Model file for the job. Use its own axes, mm. A direction names the side the tool comes from. Round coordinates to 2 decimals unless told otherwise and drop trailing zeros. Write each loop counter-clockwise with the first axis right and the second up, starting at its lowest first coordinate (ties: lowest second). Pieces come first, ordered by that corner, then holes. Notation, with made-up numbers: (25.25, -27.75) - (66.25, -27.75) arc R29 cw to (66.25, 6.25) - close; hole circle Ø8 at (-11.5, 3). An arc over 180 degrees is marked (long way). One line per item, written item: value.
Autodesk Inventor part; units mm, degrees
ref_plane "Arbeitsebene2" through (4.7579, -7.132, 2.2) normal (0, 0, 1) x (1, 0, 0)
ref_plane "YZ Plane" through (0, 0, 0) normal (1, 0, 0) x (0, 1, 0)
ref_plane "XZ Plane" through (0, 0, 0) normal (0, 1, 0) x (-1, 0, 0)
ref_plane "Arbeitsebene1" through (0, 0, 0) normal (0, 0, 1) x (1, 0, 0)
sketch "Skizze1" plane through (0, 0, 0) normal (0, 0, 1) x (1, 0, 0)
  circle A0 centre (-0.0001, 0.0021) radius 3
  circle A1 centre (11, 0) radius 2.566
  circle A2 centre (-9.5, -11) radius 1.352
  arc A3 (19, -13.5) -> (20, -12.5) centre (19, -12.5) ccw
  line L0 (20, -12.5) -> (20, 12.5)
  arc A4 (20, 12.5) -> (19, 13.5) centre (19, 12.5) ccw
  line L1 (19, 13.5) -> (-19, 13.5)
  arc A5 (-19, 13.5) -> (-20, 12.5) centre (-19, 12.5) ccw
  line L2 (-20, 12.5) -> (-20, -12.5)
  arc A6 (-20, -12.5) -> (-19, -13.5) centre (-19, -12.5) ccw
  line L3 (-19, -13.5) -> (19, -13.5)
  line L4 (18.6579, -7.132) -> (11.0758, -7.132)
  line L5 (18.6579, -7.132) -> (18.6579, 2.268)
  line L6 (18.6579, 2.268) -> (19.6579, 4.268)
  line L7 (19.6579, 4.268) -> (19.6579, 7.668)
  line L8 (18.0704, 7.668) -> (19.6579, 7.668)
  line L9 (18.0704, 7.668) -> (18.0704, 6.818)
  line L10 (18.0704, 6.818) -> (13.4704, 6.818)
  line L11 (13.4704, 6.818) -> (13.4704, 5.418)
  line L12 (13.4704, 5.418) -> (14.8704, 5.418)
  line L13 (14.8704, 5.418) -> (15.4704, 6.018)
  line L14 (15.4704, 6.018) -> (18.0704, 6.018)
  line L15 (18.0704, 6.018) -> (18.0704, 5.768)
  line L16 (18.0704, 5.768) -> (15.5704, 5.768)
  line L17 (15.5704, 5.768) -> (15.0704, 5.268)
  line L18 (15.0704, 5.268) -> (13.0704, 5.268)
  line L19 (13.0704, 5.268) -> (13.0704, 7.668)
  line L20 (6.4079, 7.668) -> (13.0704, 7.668)
  line L21 (6.4079, 7.668) -> (6.4079, 6.468)
  line L22 (4.7579, 6.468) -> (6.4079, 6.468)
  line L23 (4.7579, -7.132) -> (4.7579, 6.468)
  line L24 (5.4458, -7.132) -> (4.7579, -7.132)
  line L25 (5.4458, -7.132) -> (5.4458, -6.382)
  line L26 (5.4458, -6.382) -> (11.0758, -6.382)
  line L27 (11.0758, -6.382) -> (11.0758, -7.132)
  line L28 (9.0327, 10.168) -> (-5.2421, 10.168)
  line L29 (-5.2421, 10.168) -> (-5.2421, 8.168)
  line L30 (-5.2421, 8.168) -> (9.0327, 8.168)
  line L31 (9.0327, 8.168) -> (9.0327, 10.168)
  line L32 (-5.2421, 8.168) -> (4.7579, 8.168)
  line L33 (4.7579, 8.168) -> (4.7579, -9.632)
  line L34 (4.7579, -9.632) -> (-5.2421, -9.632)
  line L35 (-5.2421, -9.632) -> (-5.2421, 8.168)
  line L36 (4.7579, -9.632) -> (9.0327, -9.632)
  line L37 (9.0327, -9.632) -> (9.0327, -7.632)
  line L38 (9.0327, -7.632) -> (4.7579, -7.632)
  line L39 (4.7579, -7.632) -> (4.7579, -9.632)
  point P0 (0, 0)
  point P1 (4.7579, 8.168)
  dimension "d0" = 0
  dimension "d1" = 0.5
  dimension "d2" = 0.5
  dimension "d3" = 2
  dimension "d4" = 2
  dimension "d5" = 10
ref_plane "Arbeitsebene2" through (4.7579, -7.132, 2.2) normal (0, 0, 1) x (1, 0, 0)
extrude "Extrusion1" add sketch "Skizze1" along normal up to surface (2.2 mm away) contours A0 | L33 L34 L35 L30 L23 | L38 L37 L36 L33 | L30 L29 L28 L31
sketch "Skizze2" plane through (-5.2421, 10.168, 2.2) normal (0, 0, 1) x (1, 0, 0)
  line L0 (0, 0) -> (14.2747, 0)
  line L1 (0, -19.8) -> (0, 0)
  line L2 (14.2747, -19.8) -> (0, -19.8)
  line L3 (14.2747, -17.8) -> (14.2747, -19.8)
  line L4 (10, -17.8) -> (14.2747, -17.8)
  line L5 (10, -2) -> (10, -17.8)
  line L6 (14.2747, -2) -> (10, -2)
  line L7 (14.2747, 0) -> (14.2747, -2)
  line L8 (14.2747, 0) -> (0, 0)
  line L9 (14.2747, 0) -> (0, 0)
  line L10 (0, 0) -> (0, -19.8)
  line L11 (0, -19.8) -> (14.2747, -19.8)
  line L12 (14.2747, -19.8) -> (14.2747, 0)
  line L13 (9.6421, -14.568) -> (0.8421, -14.568)
  line L14 (0.8421, -14.568) -> (0.8421, -5.768)
  line L15 (0.8421, -5.768) -> (9.6421, -5.768)
  line L16 (9.6421, -5.768) -> (9.6421, -14.568)
  line L17 (9.6421, -14.568) -> (0.8421, -5.768) construction
  line L18 (0.8421, -14.568) -> (9.6421, -5.768) construction
  line L19 (0, 0) -> (0, -19.8)
  line L20 (0.8421, -5.768) -> (0, -5.768)
  line L21 (0, -5.768) -> (0, -14.568)
  line L22 (0, -14.568) -> (0.8421, -14.568)
  line L23 (0.8421, -14.568) -> (0.8421, -5.768)
  point P0 (5.2421, -10.168)
  point P1 (0, -5.768)
  point P2 (0.8421, -14.568)
  point P3 (14.2747, -17.8)
  point P4 (14.2747, -2)
  dimension "d8" = 8.8
  dimension "d9" = 8.8
extrude "Extrusion2" add sketch "Skizze2" along normal blind 2 contours L0 L7 L6 L5 L4 L3 L2 L1 L22 L13 L16 L15 L20 | L12 L4 L5 L6
sketch "Skizze3" plane through (0, 0, 0) normal (0, 0, -1) x (-1, 0, 0)
  line L0 (5.2421, 10.168) -> (5.2421, -9.632)
  line L1 (-9.0327, 10.168) -> (5.2421, 10.168)
  line L2 (-9.0327, 8.168) -> (-9.0327, 10.168)
  line L3 (-4.7579, 8.168) -> (-9.0327, 8.168)
  line L4 (-4.7579, -7.632) -> (-4.7579, 8.168)
  line L5 (-9.0327, -7.632) -> (-4.7579, -7.632)
  line L6 (-9.0327, -9.632) -> (-9.0327, -7.632)
  line L7 (5.2421, -9.632) -> (-9.0327, -9.632)
  line L8 (2.2421, -9.8367) -> (9.0217, -9.8367)
  line L9 (9.0217, -9.8367) -> (9.0217, 10.4786)
  line L10 (9.0217, 10.4786) -> (2.2421, 10.4786)
  line L11 (2.2421, 10.4786) -> (2.2421, -9.8367)
  line L12 (2.2421, -9.8367) -> (9.0217, 10.4786) construction
  line L13 (9.0217, -9.8367) -> (2.2421, 10.4786) construction
  point P0 (0, 0)
  point P1 (5.6319, 0.321)
  dimension "d12" = 3
extrude "Extrusion3" cut sketch "Skizze3" against normal blind 2.5 contours L1 L11 L10 L9 L8 L7 L0 | L0 L7 L11 L1
sketch "Skizze4" plane through (0, 0, 0) normal (0, 0, -1) x (-1, 0, 0)
  line L0 (2.2421, -9.632) -> (2.2421, 10.168)
  line L1 (-9.0327, 10.168) -> (2.2421, 10.168)
  line L2 (-9.0327, 8.168) -> (-9.0327, 10.168)
  line L3 (-4.7579, 8.168) -> (-9.0327, 8.168)
  line L4 (-4.7579, -7.632) -> (-4.7579, 8.168)
  line L5 (-9.0327, -7.632) -> (-4.7579, -7.632)
  line L6 (-9.0327, -9.632) -> (-9.0327, -7.632)
  line L7 (2.2421, -9.632) -> (-9.0327, -9.632)
  line L8 (2.2421, 4.4) -> (2.2421, 10.168)
  line L9 (2.2421, 9.168) -> (-1.1963, 9.168)
  line L10 (-1.1963, 9.168) -> (-1.1963, -8.632)
  line L11 (-1.1963, -8.632) -> (2.2421, -8.632)
  line L12 (2.2421, -8.632) -> (2.2421, 9.168)
  point P0 (0, 0)
  point P1 (2.2421, -8.632)
extrude "Extrusion4" cut sketch "Skizze4" against normal blind 2 contours L11 L10 L9 L0
sketch "Skizze5" plane through (4.4, -4.4, 2.2) normal (0, 0, 1) x (1, 0, 0)
  circle A0 centre (-4.4001, 4.4021) radius 3
  point P0 (-4.4, 4.4)
extrude "Extrusion5" add sketch "Skizze5" along normal blind 0.1
equation "\"d6\" = d2"
properties part number "Anglerfish_Cameraspacer"
1. Drop flat-ended pins along their axis: pin 1 (2 mm diameter, centred on x = 0.5, y = -1, fed in from +Z); pin 2 (0.6 mm diameter, centred on x = -2.5, y = -1, fed in from -Z); pin 3 (1.6 mm diameter, centred on y = 1.5, z = 3.5, fed in from -X). Give the stop position or say it passes through.
Report:
pin 1: z = 2.3
pin 2: z = 2
pin 3: x = 4.4
2. Band-saw the part on A-A on x = 6. Write the cut outline in (y, z), plus the area to 3 significant figures.
Report:
outline: (-9.63, 0) - (-7.63, 0) - (-7.63, 2.2) - (8.17, 2.2) - (8.17, 0) - (10.17, 0) - (10.17, 4.2) - (-9.63, 4.2) - close
area: 48.4 mm²
3. Wall check: probe 1 along Y at (x, z) = (0, 3.35); probe 2 along Z at (x, y) = (-3.25, -8); probe 3 along Z at (x, y) = (-2, 6.25). Give the ranges that are in metal, low to high. Write a range as [from, to].
Report:
probe 1: [-9.63, -4.4], [4.4, 10.17]
probe 2: [2.5, 4.2]
probe 3: [2, 4.2]
4. Mould opens along Y. For faces 1 (the face through (0, 0, 2.3)), 2 (the face through (9.033, 9, 1)), 3 (the face through (2, 10.168, 2)) say: released by +Y, released by -Y, zero draft, split by the parting line, or undercut.
Report:
face 1: undercut
face 2: zero draft
face 3: released by +Y
5. Band-saw the part on B-B on y = 3.5. Write the cut outline in (x, z).
Report:
outline: (-2.24, 2) - (1.2, 2) - (1.2, 0) - (4.76, 0) - (4.76, 2.2) - (9.03, 2.2) - (9.03, 4.2) - (4.4, 4.2) - (4.4, 2.2) - (-2.24, 2.2) - close
6. Band-saw the part on C-C on z = 1.25. Write the cut outline in (x, y), plus the area to 3 significant figures.
Report:
outline: (-2.24, -9.63) - (9.03, -9.63) - (9.03, -7.63) - (4.76, -7.63) - (4.76, 8.17) - (9.03, 8.17) - (9.03, 10.17) - (-2.24, 10.17) - (-2.24, 9.17) - (1.2, 9.17) - (1.2, -8.63) - (-2.24, -8.63) - close
area: 94.5 mm²
7. Band-saw the part on D-D on x = 0. Write the cut outline in (y, z).
Report:
outline: (-9.63, 0) - (-8.63, 0) - (-8.63, 2) - (9.17, 2) - (9.17, 0) - (10.17, 0) - (10.17, 4.2) - (4.4, 4.2) - (4.4, 2.2) - (3, 2.2) - (3, 2.3) - (-3, 2.3) - (-3, 2.2) - (-4.4, 2.2) - (-4.4, 4.2) - (-9.63, 4.2) - close
8. Tool access for faces 4 (the face through (9.033, -9, 1)), 5 (the face through (0, 4.4, 3)), 6 (the face through (7, -7.632, 1)), 7 (the face through (0, 0, 2)), 8 (the face through (-5.242, -7, 3)): list every direction of +Z, -Z, +X, -X, +Y, -Y with a clear straight run to the whole face (end or side of a thin tool).
Report:
face 4: +Z, -Z, +X, +Y, -Y
face 5: +Z, -X
face 6: -Z, +X
face 7: -Z, -X
face 8: +Z, -Z, -X, +Y, -Y
